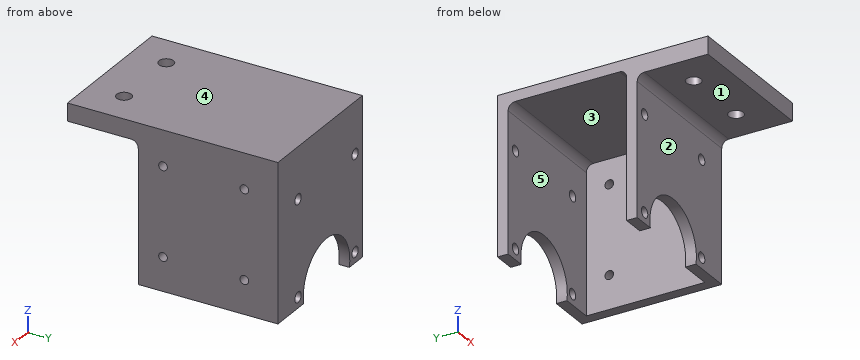
Autodesk Inventor part; units mm, degrees
ref_plane "YZ Plane" through (0, 0, 0) normal (1, 0, 0) x (0, 1, 0)
ref_plane "XZ Plane" through (0, 0, 0) normal (0, 1, 0) x (-1, 0, 0)
ref_plane "XY Plane" through (0, 0, 0) normal (0, 0, 1) x (1, 0, 0)
sketch "スケッチ1" plane through (0, 0, 0) normal (0, 1, 0) x (-1, 0, 0)
  line L0 (0, 0) -> (-34, 0)
  line L1 (-34, 0) -> (-34, -44.5)
  line L2 (-34, -44.5) -> (0, -44.5)
  line L3 (0, -44.5) -> (0, 0)
  dimension "d0" = 44.5
  dimension "d1" = 34
extrude "押し出し1" add sketch "スケッチ1" along normal blind 39.5
sketch "スケッチ2" plane through (34, 0, 0) normal (1, 0, 0) x (0, 0, -1)
  line L0 (3, 36.5) -> (53, 36.5)
  line L1 (53, 36.5) -> (53, 3)
  line L2 (53, 3) -> (3, 3)
  line L3 (3, 3) -> (3, 36.5)
  line L4 (0, 39.5) -> (44.5, 39.5)
  line L5 (0, 0) -> (0, 39.5)
  dimension "d4" = 3
  dimension "d5" = 3
  dimension "d6" = 33.5
  dimension "d7" = 50
extrude "押し出し2" cut sketch "スケッチ2" against normal blind 43.5
sketch "スケッチ3" plane through (0, 0, 0) normal (0, -1, 0) x (1, 0, 0)
  circle A0 centre (17, -42.5) radius 11
  line L0 (34, -44.5) -> (0, -44.5)
  line L1 (0, -44.5) -> (0, 0)
  point P0 (6.1833, -44.5)
  point P1 (27.8167, -44.5)
  dimension "d10" = 22
  dimension "d11" = 2
  dimension "d12" = 17
extrude "押し出し3" cut sketch "スケッチ3" against normal blind 3 contours A0 L0 picked at (20.7405, -38.2254)
sketch "スケッチ4" plane through (0, 39.5, 0) normal (0, 1, 0) x (1, 0, 0)
  circle A0 centre (17, 42.5) radius 11
  line L0 (34, 44.5) -> (0, 44.5)
  line L1 (0, 44.5) -> (0, 0)
  point P0 (27.8167, 44.5)
  point P1 (6.1833, 44.5)
  point P2 (0, 35.0774)
  dimension "d15" = 22
  dimension "d16" = 2
  dimension "d17" = 17
extrude "押し出し4" cut sketch "スケッチ4" against normal blind 3
sketch "スケッチ5" plane through (0, 39.5, 0) normal (0, 1, 0) x (1, 0, 0)
  line L0 (0, 0) -> (34, 0)
  line L1 (0, 44.5) -> (0, 0)
  line L2 (34, 0) -> (34, 44.5)
  point P0 (3.5, 14.5)
  point P1 (3.5, 41.5)
  point P2 (30.5, 41.5)
  point P3 (30.5, 14.5)
  dimension "d20" = 14.5
  dimension "d21" = 3.5
  dimension "d22" = 27
  dimension "d23" = 3.5
  dimension "d48" = 3.5
  dimension "d55" = 14.5
  dimension "d56" = 27
hole "穴1" at (3.5, 39.5, -14.5) at (3.5, 39.5, -41.5) at (30.5, 39.5, -41.5) at (30.5, 39.5, -14.5) direction (0, -1, 0) diameter 3 end through all
fillet "フィレット1" radius 2 1 edges at (17, 36.5, -3)
fillet "フィレット2" radius 2 1 edges at (17, 3, -3)
sketch "スケッチ8" plane through (0, 0, 0) normal (0, 0, 1) x (1, 0, 0)
  line L0 (0, 0) -> (34, 0)
  line L1 (34, 0) -> (34, -20)
  line L2 (34, -20) -> (0, -20)
  line L3 (0, -20) -> (0, 0)
  line L4 (34, 0) -> (34, 39.5)
  dimension "d59" = 20
extrude "押し出し5" add sketch "スケッチ8" against normal blind 5
sketch "スケッチ9" plane through (0, 0, -5) normal (0, 0, -1) x (-1, 0, 0)
  line L0 (-30, -10) -> (-10, -10)
  line L1 (-34, -20) -> (0, -20)
  line L2 (-34, 0) -> (-34, -20)
  line L3 (0, -20) -> (0, 0)
  point P0 (-17, -20)
  point P1 (-34, -10)
  dimension "d62" = 20
  dimension "d71" = 10
hole "穴3" at (30, -10, -5) at (10, -10, -5) direction (0, 0, 1) diameter 4.134 end through all
sketch "スケッチ11" plane through (34, 39.5, 0) normal (1, 0, 0) x (0, 0, -1)
  line L0 (3, -34.5) -> (3, -5)
  arc A0 (5, -3) -> (3, -5) centre (5, -5) ccw
  line L1 (5, -3) -> (44.5, -3)
  line L2 (44.5, -3) -> (44.5, 0)
  line L3 (0, 0) -> (44.5, 0)
  line L4 (0, -59.5) -> (0, 0)
  line L5 (0, -59.5) -> (5, -59.5)
  line L6 (5, -39.5) -> (5, -59.5)
  line L7 (44.5, -36.5) -> (5, -36.5)
  arc A1 (3, -34.5) -> (5, -36.5) centre (5, -34.5) ccw
  line L8 (5, -39.5) -> (44.5, -39.5)
  line L9 (44.5, -39.5) -> (44.5, -36.5)
  point P0 (0, -39.5)
extrude "押し出し6" add sketch "スケッチ11" along normal blind 6
fillet "フィレット4" radius 2 1 edges at (20, 0, -5)
sketch "スケッチ17" plane through (40, 39.5, 0) normal (1, 0, 0) x (0, 0, -1)
  line L0 (44.5, -36.5) -> (5, -36.5)
  line L1 (44.5, -36.5) -> (3, -36.5)
  line L2 (3, -36.5) -> (3, -3)
  line L3 (3, -3) -> (44.5, -3)
  line L4 (44.5, -3) -> (44.5, -36.5)
  point P0 (0, -39.5)
  point P1 (5, -36.5)
extrude "押し出し9" add sketch "スケッチ17" against normal blind 3
sketch "スケッチ19" plane through (40, 39.5, 0) normal (1, 0, 0) x (0, 0, -1)
  line L0 (44.5, 0) -> (0, 0)
  line L1 (0, 0) -> (0, -59.5)
  point P0 (0, -39.5)
  point P1 (10, -9.5)
  point P2 (35, -9.5)
  point P3 (10, -32.5)
  point P4 (35, -32.5)
  dimension "d114" = 9.5
  dimension "d115" = 10
  dimension "d118" = 25
  dimension "d125" = 23
  dimension "d137" = 23
hole "穴6" at (40, 30, -10) at (40, 30, -35) at (40, 7, -10) at (40, 7, -35) direction (-1, 0, 0) diameter 2.459 end through all
properties part number "サーボモータ固定用"
Geometry: final body of the model. Coordinates: model frame, mm. Face numbers are marked on the shaded views. A direction names the side the tool comes from. Coordinates: 2 decimals unless noted, no trailing zeros. Loops run counter-clockwise (first coordinate to the right, second up) from the corner with the lowest first, then second, coordinate; pieces in that order, holes last. Notation, with made-up numbers: (-7.5, 56.25) - (5.5, 56.25) arc R19 cw to (5.5, 66.25) - close; hole circle Ø10 at (31.25, 12). An arc over 180 degrees is marked (long way). One line per question, with ' | ' between items. Start each with the question number.
(1) Cut plane C-C on y = 7. Output: boundary loops of the cut face in (x, z), and give its area (3 significant figures).
(2) Reachability of the marked faces 4 and 5 from +Z, -Z, +X, -X, +Y, -Y: full face, straight path, thin tool, end or side. Return the list, or none.
(3) Draft query along Y for the marked faces 1, 2 and 3. Return one class per face: +Y half, -Y half, draft (parallel to the pull), parting line (faces both ways), or undercut.
(4) Cut plane B-B on z = -24. Output: boundary loops of the cut face in (x, y), and give its area (4 significant figures).
(5) Cut plane D-D on x = 10. Output: boundary loops of the cut face in (y, z).
(6) First-contact query: pin 1 (6 mm diameter, centred on x = 14.5, y = 15, fed in from -Z); pin 2 (5 mm diameter, centred on x = 10, y = -10, fed in from +Z); pin 3 (5.5 mm diameter, centred on x = 21, y = -9, fed in from -Z); pin 4 (3 mm diameter, centred on y = 30, z = -35, fed in from -X). Flat tips, straight axial feed; report the tip coordinate or a pass-through.
(7) Ray query, L1, parallel to Z at x = 38, y = 7; L2, parallel to Y at x = 27.5, z = -13; L3, parallel to X at y = 37.5, z = -14.5. Return the intervals inside material, ascending. Write a range as from..to.
(8) Cut plane A-A on x = 3.5. Count the separate pieces of the cut face and the enclosed holes in it, and give its area (3 significant figures).
Here are the results:
1) outline: (0, -3) - (37, -3) - (37, -8.77) - (40, -8.77) - (40, 0) - (0, 0) - close; (37, -44.5) - (40, -44.5) - (40, -36.23) - (37, -36.23) - close; (37, -33.77) - (40, -33.77) - (40, -11.23) - (37, -11.23) - close | area: 230 mm²
2) face 4: +Z, +X, -X, +Y, -Y | face 5: -Z, -X
3) face 1: draft | face 2: -Y half | face 3: undercut
4) outline: (0, 0) - (40, 0) - (40, 39.5) - (0, 39.5) - (0, 36.5) - (37, 36.5) - (37, 3) - (0, 3) - close | area: 340.5 mm²
5) outline: (-20, -5) - (-12.07, -5) - (-12.07, 0) - (-20, 0) - close; (-7.93, -5) - (-2, -5) arc R2 cw to (0, -7) - (0, -34.01) - (3, -34.01) - (3, -5) arc R2 cw to (5, -3) - (34.5, -3) arc R2 cw to (36.5, -5) - (36.5, -34.01) - (39.5, -34.01) - (39.5, 0) - (-7.93, 0) - close
6) pin 1: z = -3 | pin 2: z = 0 | pin 3: z = -5 | pin 4: x = 37
7) L1: -44.5..-36.23, -33.77..-11.23, -8.77..0 | L2: 0..3, 36.5..39.5 | L3: 0..2, 5..29, 32..40
8) separate pieces: 5 | enclosed holes: 0 | area: 434 mm²
